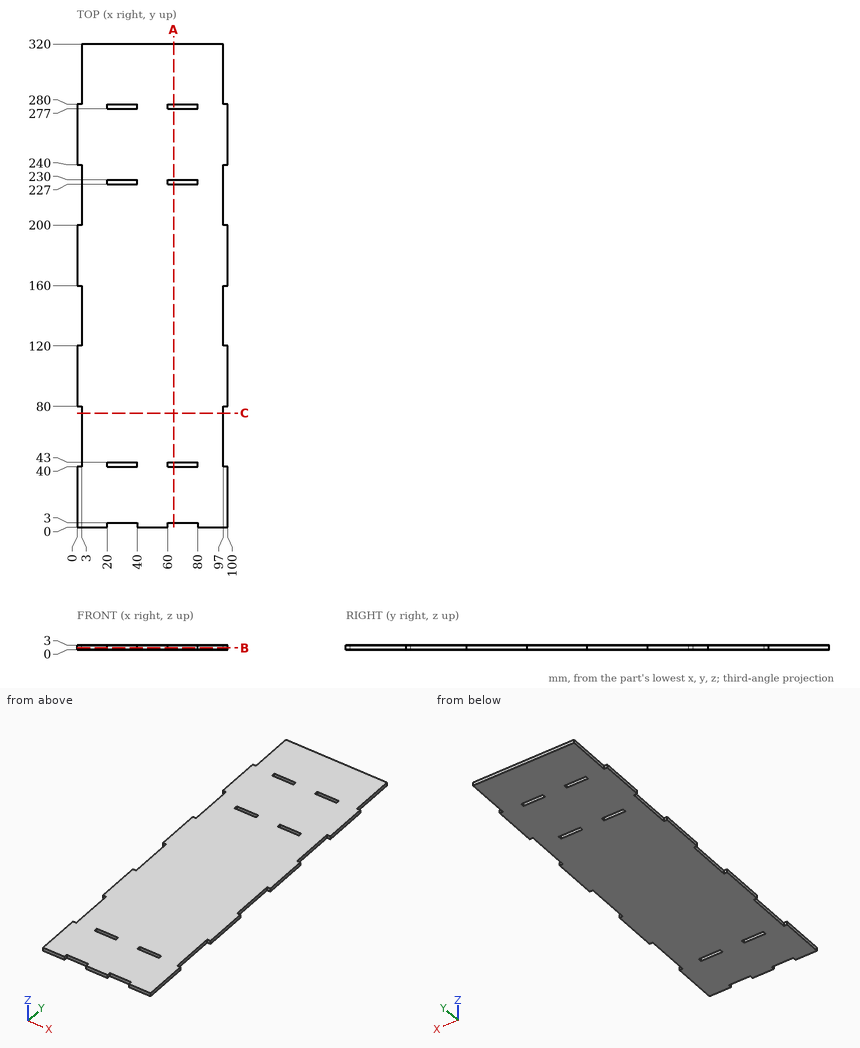
Here's the drawing with two shaded views (mm, measured from the low corner). I have some questions. Coordinates: 2 decimals unless noted, no trailing zeros. Loops run counter-clockwise (first coordinate to the right, second up) from the corner with the lowest first, then second, coordinate; pieces in that order, holes last. Notation, with made-up numbers: M 32,69 L 68,69 A12 cw 68,77 Z; hole C 42.5,-32 d11. An arc over 180 degrees is marked long. Answer as CSV lines item,"result". Start each with the question number.
1. Suppose I cut it at A-A, the plane x = 64. List the corners of the cut face in (y, z) for me.
2. Suppose I cut it at B-B, the plane z = 1.2. Count the separate pieces of the cut face and the enclosed holes in it, plus the area to 3 significant figures.
3. Suppose I cut it at C-C, the plane y = 75.5. List the corners of the cut face in (x, z) for me.
4. For pin 1 Ø1.5 at (x, z) = (99, 2) entering from +Y; pin 2 Ø0.9 at (y, z) = (41, 1.5) entering from +X; pin 3 Ø1 at (y, z) = (136, 1.5) entering from -X, each with a flat end and sliding along its axis, tell me the tip position at first contact or that it passes through.
5. If I drill on probe 1 along Y at (x, z) = (76, 2.45); probe 2 along X at (y, z) = (42.5, 1.5); probe 3 along X at (y, z) = (78, 0.2), over which ranges is the centre line in solid material (lowest first)? Write a range as [from, to].
Output:
1,outline,"M 3,0 L 40,0 L 40,3 L 3,3 Z; M 43,0 L 227,0 L 227,3 L 43,3 Z; M 230,0 L 277,0 L 277,3 L 230,3 Z; M 280,0 L 320,0 L 320,3 L 280,3 Z"
2,separate pieces,"1"
2,enclosed holes,"6"
2,area,"30,600 mm^2"
3,outline,"M 3,0 L 97,0 L 97,3 L 3,3 Z"
4,pin 1,"stops at y = 280"
4,pin 2,"stops at x = 97"
4,pin 3,"stops at x = 3"
5,probe 1,"y = [3, 40], [43, 227], [230, 277], [280, 320]"
5,probe 2,"x = [3, 20], [40, 60], [80, 97]"
5,probe 3,"x = [3, 97]"
